```python
from build123d import *

# Parameters (mm, degrees)
SKETCH_1_W          = 12
SKETCH_1_H          = 11
EXTRUDE_1_DEPTH     = 2
CUT_EXTRUDE_2_DEPTH = 2


with BuildPart() as part:
    # 草图1 → 凸台-拉伸1 (new body)
    with BuildSketch(Plane.XY):
        with Locations((-0.010267275, -0.272881356)):
            Rectangle(SKETCH_1_W, SKETCH_1_H)
    extrude(amount=EXTRUDE_1_DEPTH)

    # 草图2 → 切除-拉伸2 (cut)
    with BuildSketch(Plane.XY.offset(2)):
        with BuildLine():
            Line((0, 1), (-1.732050808, 1))
            ThreePointArc((-1.732050808, 1), (-0.51763809, -1.931851653), (2, 0))
            ThreePointArc((2, 0), (1.931851653, 0.51763809), (1.732050808, 1))
            Line((1.732050808, 1), (0, 1))
        make_face()
    extrude(amount=-CUT_EXTRUDE_2_DEPTH, mode=Mode.SUBTRACT)


solid = part.part
```
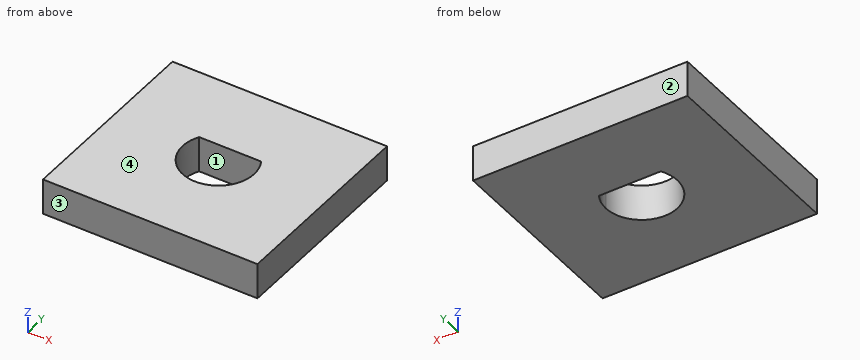
Input: part model. Units: mm. Frame: model coordinates. Face numbers are marked on the shaded views. Give positions to 0.01 mm unless a question says otherwise; leave off trailing zeros. Order: outer loops, then holes, each group sorted by start corner. A loop starts at its lowest first (then second) coordinate and runs counter-clockwise, first axis right, second up. Notation, with made-up numbers: M 68,53.5 L 124,53.5 A14 ccw 124,70.5 Z; hole C 35.25,34 d9. An arc over 180 degrees is marked long. One line per question, with ' | ' between items.
1) Section A-A on x = 0. Output: boundary loops of the cut face in (y, z), and give its area (3 significant figures).
Filled in:
outline: M -5.77,0 L -2,0 L -2,2 L -5.77,2 Z; M 1,0 L 5.23,0 L 5.23,2 L 1,2 Z | area: 16.0 mm2
2) Section B-B on z = 0.9. Output: boundary loops of the cut face in (x, y).
Filled in:
outline: M -6.01,-5.77 L 5.99,-5.77 L 5.99,5.23 L -6.01,5.23 Z; hole M -1.73,1 A2 ccw long 1.73,1 Z
3) Ray query, L1, parallel to Y at x = 0, z = 0.8; L2, parallel to Y at x = 1, z = 1.5; L3, parallel to X at y = 0, z = 1.35. Return the intervals inside material, ascending.
Filled in:
L1: y = -5.77 to -2, 1 to 5.23 | L2: y = -5.77 to -1.73, 1 to 5.23 | L3: x = -6.01 to -2, 2 to 5.99
4) Section C-C on y = -0.75. Output: boundary loops of the cut face in (x, z), and give its area (3 significant figures).
Filled in:
outline: M -6.01,0 L -1.85,0 L -1.85,2 L -6.01,2 Z; M 1.85,0 L 5.99,0 L 5.99,2 L 1.85,2 Z | area: 16.6 mm2
5) Draft query along Y for the marked faces 1, 2, 3 and 4. Return one class per face: pulls with the +Y half, pulls with the -Y half, needs draft (parallel to the pull), parting line crosses it, or undercut.
Filled in:
face 1: undercut | face 2: pulls with the +Y half | face 3: pulls with the -Y half | face 4: needs draft
